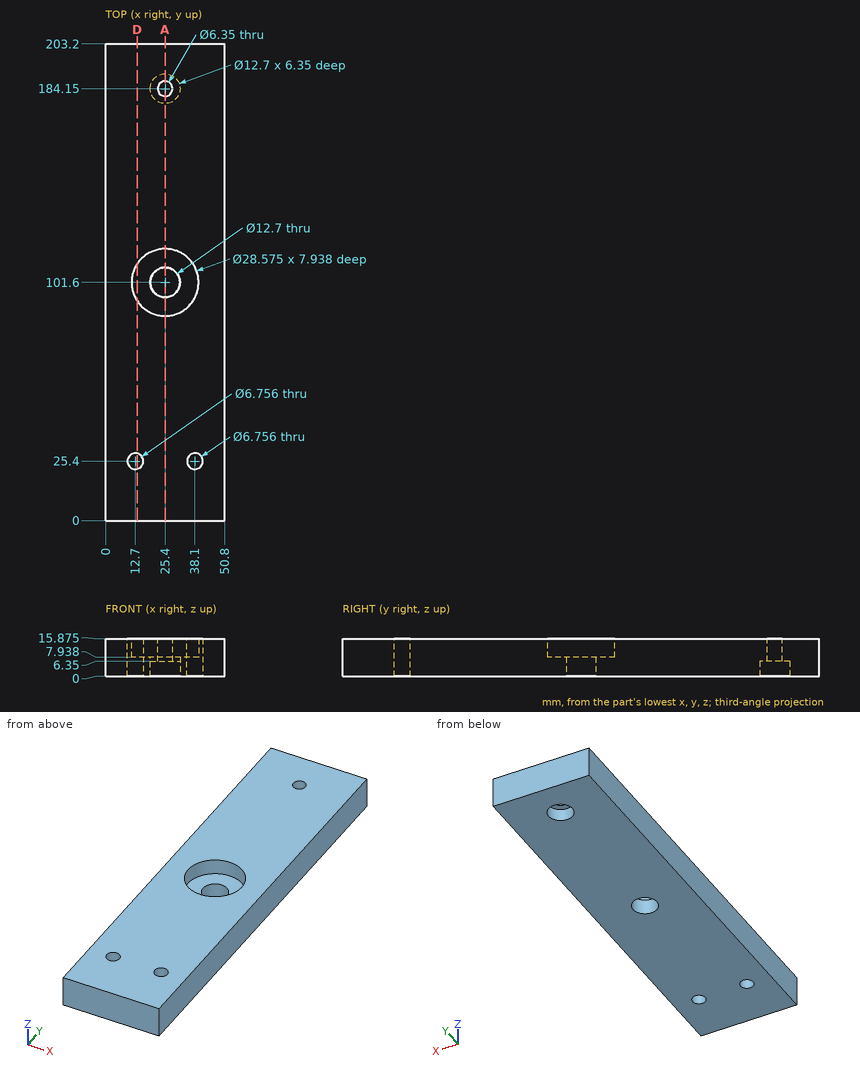
Verification items for this drawing (mm, ordinates from the low corner). Coordinates: 2 decimals unless noted, no trailing zeros. Order: outer loops, then holes, each group sorted by start corner. A loop starts at its lowest first (then second) coordinate and runs counter-clockwise, first axis right, second up.
Q1. Sectioned sample at A-A on x = 25.4. Give the number of separate pieces and of enclosed holes in the cut face, and give its area (3 significant figures).
Reply:
separate pieces: 3
enclosed holes: 0
area: 2,760 mm2
Q2. Thickness scan on probe 1 along Y at (x, z) = (25.4, 13) (1 decimal); probe 2 along Y at (x, z) = (26, 3); probe 3 along X at (y, z) = (184.15, 13) (1 decimal). Record the ranges inside material, lowest first.
Reply:
probe 1: y = 0 to 87.3, 115.9 to 181, 187.3 to 203.2
probe 2: y = 0 to 95.28, 107.92 to 177.83, 190.47 to 203.2
probe 3: x = 0 to 22.2, 28.6 to 50.8
Q3. Sectioned sample at D-D on x = 13.5. Record the cut outline in (y, z) (1 decimal), and give its area (3 significant figures).
Reply:
outline: (0, 0) - (22.1, 0) - (22.1, 15.9) - (0, 15.9) - close; (28.7, 0) - (203.2, 0) - (203.2, 15.9) - (109.5, 15.9) - (109.5, 7.9) - (93.7, 7.9) - (93.7, 15.9) - (28.7, 15.9) - close
area: 3,000 mm2
Q4. Depth check by flat-ended pin: pin 1 Ø8.5 at (x, y) = (25.4, 184.15) entering from -Z. Enter the tip coordinate at first touch or a pass-through.
Reply:
pin 1: stops at z = 6.35
